For this review, take the finished solid that the model builds, in its own axes (mm). A direction names the side the tool comes from. Round coordinates to 2 decimals unless told otherwise and drop trailing zeros. Write each loop counter-clockwise with the first axis right and the second up, starting at its lowest first coordinate (ties: lowest second). Pieces come first, ordered by that corner, then holes. Notation, with made-up numbers: (69, -9.75) - (111, -9.75) arc R37 cw to (111, 28.25) - close; hole circle Ø3 at (6, 59). An arc over 180 degrees is marked (long way). One line per item, written item: value. Start each with the question number.
Q1. Add section A-A on x = 18. Write out the cut boundary in (y, z).
Q2. Add section D-D on y = 36. Write out the cut boundary in (x, z).
Q3. Clearance check with flat-ended pins moving along their axes: pin 1 Ø5 at (y, z) = (30, 15) entering from +X; pin 2 Ø5 at (x, y) = (14, 37) entering from +Z; pin 3 Ø10 at (y, z) = (5, 30.5) entering from +X; pin 4 Ø16 at (x, y) = (40, 20) entering from +Z. State where each tip first meets the part, or that it passes through.
Q4. For probe 1 along Y at (x, z) = (40, 7.25); probe 2 along Z at (x, y) = (41, 9.5), list the stretches that pass through material, from the lowest coordinate up.
Q5. Add section C-C on y = 11.5. Write out the cut boundary in (x, z).
Q6. Mouldability with a two-part tool opening along Y and no side actions: class faces 1 (the face through (11, 40, 15)), 2 (the face through (38.698, 29.915, 4.93)), 3 (the face through (15, 5, 20)) as +Y half, -Y half, draft (parallel to the pull), parting line (faces both ways), or undercut.
Q7. Tool access review of faces 4 (the face through (0, 15, 11)), 5 (the face through (10, 20, 32)): name each direction out of +Z, -Z, +X, -X, +Y, -Y from which nothing blocks a thin tool from reaching the whole face with its end or side.
Q8. Add section B-B on z = 23.5. Write out the cut boundary in (x, y), and give its area (3 significant figures).
```python
from build123d import *

# Parameters (mm, degrees)
F0_W     = 10
F0_H     = 40
F1_DEPTH = 40
F2_DEPTH = 20
F0_R     = 10
F3_DEPTH = 10
F5_DEPTH = 20.001


with BuildPart() as f1:
    # F0 (on Top) → F1 (new body)
    with BuildSketch(Plane.XY):
        with Locations((5, 20)):
            Rectangle(F0_W, F0_H)
    extrude(amount=F1_DEPTH)

    # F0 (on Top) → F2 (join)
    with BuildSketch(Plane.XY):
        with Locations((15, 20)):
            Rectangle(F0_W, F0_H)
    extrude(amount=F2_DEPTH)

    # F0 (on Top) → F3 (join)
    with BuildSketch(Plane.XY):
        with BuildLine():
            Line((20, 40), (20, 0))
            Line((20, 0), (40, 0))
            ThreePointArc((40, 0), (60, 20), (40, 40))
            Line((40, 40), (20, 40))
        make_face()
        with Locations((40, 20)):
            Circle(F0_R, mode=Mode.SUBTRACT)
    extrude(amount=F3_DEPTH)

    # F4 (on face) → F5 (cut, through all)
    with BuildSketch(Plane.YZ.offset(20)):
        with BuildLine():
            ThreePointArc((20, 10), (27.071068, 12.928932), (30, 20))
            Line((30, 20), (10, 20))
            ThreePointArc((10, 20), (12.928932, 12.928932), (20, 10))
        make_face()
        with BuildLine():
            Line((10, 20), (30, 20))
            ThreePointArc((30, 20), (20, 30), (10, 20))
        make_face()
    extrude(amount=-F5_DEPTH, mode=Mode.SUBTRACT)


solid = f1.part
```
Result set:
1. outline: (0, 0) - (40, 0) - (40, 20) - (30, 20) arc R10 cw to (20, 10) arc R10 cw to (10, 20) - (0, 20) - close
2. outline: (0, 0) - (52, 0) - (52, 10) - (20, 10) - (20, 20) - (10, 20) - (10, 40) - (0, 40) - close
3. pin 1: stops at x = 20
3. pin 2: stops at z = 20
3. pin 3: stops at x = 10
3. pin 4: passes through
4. probe 1: y = 0 to 10, 30 to 40
4. probe 2: z = 0 to 10
5. outline: (0, 0) - (34.73, 0) - (34.73, 10) - (20, 10) - (20, 14.73) - (0, 14.73) - close; (0, 25.27) - (10, 25.27) - (10, 40) - (0, 40) - close; (45.27, 0) - (58.1, 0) - (58.1, 10) - (45.27, 10) - close
6. face 1: +Y half
6. face 2: undercut
6. face 3: draft
7. face 4: +Z, -Z, -X, +Y, -Y
7. face 5: +Z, +X, +Y, -Y
8. outline: (0, 0) - (10, 0) - (10, 10.63) - (0, 10.63) - close; (0, 29.37) - (10, 29.37) - (10, 40) - (0, 40) - close
8. area: 213 mm^2
